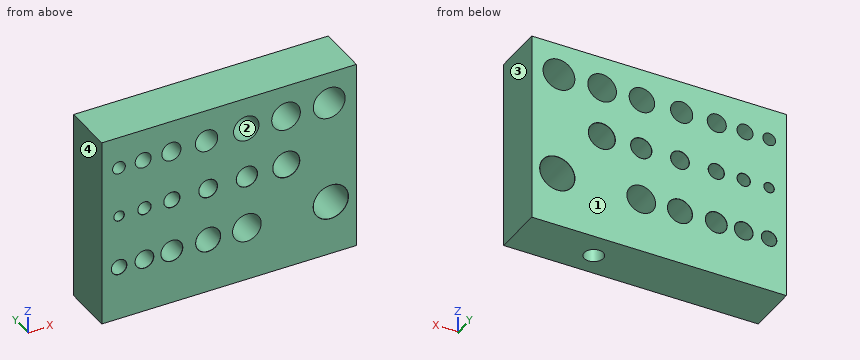
from build123d import *

# Parameters (mm, degrees)
SKETCH1_W            = 40
SKETCH1_H            = 30
SKETCH1_R            = 1
SKETCH1_R_2          = 1.25
SKETCH1_R_3          = 1.5
SKETCH1_R_4          = 1.75
SKETCH1_R_5          = 2
SKETCH1_R_6          = 2.25
SKETCH1_R_7          = 2.5
BOSS_EXTRUDE1_DEPTH  = 8
M4_CLEARANCE_HOLE1_D = 4.5
SKETCH27_R           = 1.5
CUT_EXTRUDE1_DEPTH   = 5


with BuildPart() as part:
    # Sketch1 → Boss-Extrude1 (new body)
    with BuildSketch(Plane(origin=(0, 0, 0), x_dir=(1, 0, 0), z_dir=(0, 1, 0))):
        with Locations((20, 15)):
            Rectangle(SKETCH1_W, SKETCH1_H)
        with Locations(Location((2.702313996, 5, 0), (0, 0, 270))):
            Circle(SKETCH1_R, mode=Mode.SUBTRACT)
        with Locations(Location((6.502577789, 5, 0), (0, 0, 270))):
            Circle(SKETCH1_R_2, mode=Mode.SUBTRACT)
        with Locations(Location((10.936495054, 5, 0), (0, 0, 270))):
            Circle(SKETCH1_R_3, mode=Mode.SUBTRACT)
        with Locations(Location((16.456979767, 5, 0), (0, 0, 270))):
            Circle(SKETCH1_R_4, mode=Mode.SUBTRACT)
        with Locations(Location((22.700422461, 5, 0), (0, 0, 270))):
            Circle(SKETCH1_R_5, mode=Mode.SUBTRACT)
        with Locations(Location((28.945995634, 5, 0), (0, 0, 270))):
            Circle(SKETCH1_R_6, mode=Mode.SUBTRACT)
        with Locations(Location((35.732366972, 5, 0), (0, 0, 270))):
            Circle(SKETCH1_R_7, mode=Mode.SUBTRACT)
    extrude(amount=BOSS_EXTRUDE1_DEPTH)

    # Sketch4 → Tap Drill for M2x0.4 Tap1 (revolve, cut)
    with BuildSketch(Plane(origin=(2.720220683, 8, -13), x_dir=(0, 0, 1), z_dir=(1, 0, 0))):
        Polygon((0, 0), (0, 8), (0.825, 8), (0.8, 7.975), (0.8, 0.025), (0.825, 0), align=None)
    revolve(axis=Axis((2.720220683, 14.35, -13), (0, -1, 0)), mode=Mode.SUBTRACT)

    # Sketch6 → Tap Drill for M2.5x0.45 Tap1 (revolve, cut)
    with BuildSketch(Plane(origin=(6.703721211, 8, -13), x_dir=(0, 0, 1), z_dir=(1, 0, 0))):
        Polygon((0, 0), (0, 8), (1.05, 8), (1.025, 7.975), (1.025, 0.025), (1.05, 0), align=None)
    revolve(axis=Axis((6.703721211, 14.35, -13), (0, -1, 0)), mode=Mode.SUBTRACT)

    # Sketch8 → Tap Drill for M3x0.5 Tap1 (revolve, cut)
    with BuildSketch(Plane(origin=(11.010208268, 8, -13), x_dir=(0, 0, 1), z_dir=(1, 0, 0))):
        Polygon((0, 0), (0, 8), (1.275, 8), (1.25, 7.975), (1.25, 0.025), (1.275, 0), align=None)
    revolve(axis=Axis((11.010208268, 14.35, -13), (0, -1, 0)), mode=Mode.SUBTRACT)

    # Sketch10 → Tap Drill for M3.5x0.6 Tap1 (revolve, cut)
    with BuildSketch(Plane(origin=(16.716303619, 8, -13), x_dir=(0, 0, 1), z_dir=(1, 0, 0))):
        Polygon((0, 0), (0, 8), (1.475, 8), (1.45, 7.975), (1.45, 0.025), (1.475, 0), align=None)
    revolve(axis=Axis((16.716303619, 14.35, -13), (0, -1, 0)), mode=Mode.SUBTRACT)

    # Sketch12 → Tap Drill for M4x0.7 Tap1 (revolve, cut)
    with BuildSketch(Plane(origin=(22.799216587, 8, -13), x_dir=(0, 0, 1), z_dir=(1, 0, 0))):
        Polygon((0, 0), (0, 8), (1.675, 8), (1.65, 7.975), (1.65, 0.025), (1.675, 0), align=None)
    revolve(axis=Axis((22.799216587, 14.35, -13), (0, -1, 0)), mode=Mode.SUBTRACT)

    # Sketch14 → Tap Drill for M5x0.8 Tap1 (revolve, cut)
    with BuildSketch(Plane(origin=(28.989791732, 8, -13), x_dir=(0, 0, 1), z_dir=(1, 0, 0))):
        Polygon((0, 0), (0, 8), (2.125, 8), (2.1, 7.975), (2.1, 0.025), (2.125, 0), align=None)
    revolve(axis=Axis((28.989791732, 14.35, -13), (0, -1, 0)), mode=Mode.SUBTRACT)

    # Sketch16 → M2 Clearance Hole1 (revolve, cut)
    with BuildSketch(Plane(origin=(2.720220683, 8, -21.453439382), x_dir=(0, 0, 1), z_dir=(1, 0, 0))):
        Polygon((0, 0), (0, 8), (1.225, 8), (1.2, 7.975), (1.2, 0.025), (1.225, 0), align=None)
    revolve(axis=Axis((2.720220683, 14.35, -21.453439382), (0, -1, 0)), mode=Mode.SUBTRACT)

    # Sketch18 → M2.5 Clearance Hole1 (revolve, cut)
    with BuildSketch(Plane(origin=(6.703721211, 8, -21.453439382), x_dir=(0, 0, 1), z_dir=(1, 0, 0))):
        Polygon((0, 0), (0, 8), (1.475, 8), (1.45, 7.975), (1.45, 0.025), (1.475, 0), align=None)
    revolve(axis=Axis((6.703721211, 14.35, -21.453439382), (0, -1, 0)), mode=Mode.SUBTRACT)

    # Sketch20 → M3 Clearance Hole1 (revolve, cut)
    with BuildSketch(Plane(origin=(11.010208268, 8, -21.453439382), x_dir=(0, 0, 1), z_dir=(1, 0, 0))):
        Polygon((0, 0), (0, 8), (1.725, 8), (1.7, 7.975), (1.7, 0.025), (1.725, 0), align=None)
    revolve(axis=Axis((11.010208268, 14.35, -21.453439382), (0, -1, 0)), mode=Mode.SUBTRACT)

    # Sketch22 → M3.5 Clearance Hole1 (revolve, cut)
    with BuildSketch(Plane(origin=(16.716303619, 8, -21.453439382), x_dir=(0, 0, 1), z_dir=(1, 0, 0))):
        Polygon((0, 0), (0, 8), (1.975, 8), (1.95, 7.975), (1.95, 0.025), (1.975, 0), align=None)
    revolve(axis=Axis((16.716303619, 14.35, -21.453439382), (0, -1, 0)), mode=Mode.SUBTRACT)

    # M4 Clearance Hole1 (through all)
    with Locations(Plane(origin=(0, 8, 0), x_dir=(1, 0, 0), z_dir=(0, 1, 0))):
        with Locations((22.799216587, 21.453439382)):
            Hole(M4_CLEARANCE_HOLE1_D / 2)

    # Sketch26 → M5 Clearance Hole1 (revolve, cut)
    with BuildSketch(Plane(origin=(35.9878332, 8, -21.453439382), x_dir=(0, 0, 1), z_dir=(1, 0, 0))):
        Polygon((0, 0), (0, 8), (2.775, 8), (2.75, 7.975), (2.75, 0.025), (2.775, 0), align=None)
    revolve(axis=Axis((35.9878332, 14.35, -21.453439382), (0, -1, 0)), mode=Mode.SUBTRACT)

    # Sketch27 → Cut-Extrude1 (cut)
    with BuildSketch(Plane(origin=(0, 0, -30), x_dir=(-1, 0, 0), z_dir=(0, 0, -1))):
        with Locations((-27.944979247, 3.833613)):
            Circle(SKETCH27_R)
    extrude(amount=-CUT_EXTRUDE1_DEPTH, mode=Mode.SUBTRACT)


solid = part.part
Input: part model. Units: mm. Frame: model coordinates. Face numbers are marked on the shaded views. Give positions to 0.01 mm unless a question says otherwise; leave off trailing zeros. Use one line per item in the form item = value. Start each with the question number.
1) Pin query (flat end, axial travel): pin 1 (0.9 mm diameter, centred on x = 27.5, y = 4, fed in from -Z). Return the tip coordinate at first contact, or that it passes through.
2) Draft query along X for the marked faces 1, 2, 3 and 4. Return one class per face: pulls with the +X half, pulls with the -X half, needs draft (parallel to the pull), parting line crosses it, or undercut.
3) Section query A-A on z = -5. Count the separate pieces of the cut face and the enclosed holes in it, then the cut area to 3 significant figures.
4) Ray query, probe 1 along Z at (x, y) = (29, 6.25); probe 2 along Z at (x, y) = (18, 0.75); probe 3 along Z at (x, y) = (3, 4.5). Return the intervals inside material, ascending. Write a range as from..to.
Outcome:
q1.pin_1 = -25
q2.face_1 = needs draft
q2.face_2 = undercut
q2.face_3 = pulls with the +X half
q2.face_4 = pulls with the -X half
q3.separate_pieces = 8
q3.enclosed_holes = 0
q3.area = 124 mm^2
q4.probe_1 = -30..-15.1, -10.9..-7.25, -2.75..0
q4.probe_2 = -30..-22.92, -19.99..-13.67, -12.33..-5.83, -4.17..0
q4.probe_3 = -30..-22.62, -20.29..-13.75, -12.25..-5.95, -4.05..0
